Autodesk Inventor part; units mm, degrees
ref_plane "YZ Plane" through (0, 0, 0) normal (1, 0, 0) x (0, 1, 0)
ref_plane "XZ Plane" through (0, 0, 0) normal (0, 1, 0) x (-1, 0, 0)
ref_plane "XY Plane" through (0, 0, 0) normal (0, 0, 1) x (1, 0, 0)
sketch "Sketch1" plane through (0, 0, 0) normal (0, 1, 0) x (-1, 0, 0)
  line L0 (75, 0) -> (-75, 0)
  line L1 (-75, 0) -> (-75, -90)
  line L2 (-75, -90) -> (75, -90)
  line L3 (75, -90) -> (75, 0)
  point P0 (0, 0)
  point P1 (0, 0)
  dimension "d0" = 150
  dimension "d1" = 90
extrude "Extrusion1" add sketch "Sketch1" along normal blind 19
sketch "Sketch2" plane through (-75, 0, 0) normal (0, 0, 1) x (1, 0, 0)
  line L0 (0, 0) -> (150, 0)
  line L1 (150, 0) -> (150, 19)
  line L2 (0, 19) -> (150, 19)
  line L3 (0, 0) -> (0, 19)
  point P0 (75, 0)
  point P1 (75, 4)
  point P2 (75, 14)
  dimension "d4" = 4
  dimension "d5" = 14
  dimension "d6" = 75
  dimension "d7" = 75
hole "Hole1" at (0, 4, 0) at (0, 14, 0) direction (0, 0, -1) diameter 3.302 depth 21
sketch "Sketch3" plane through (0, 19, 0) normal (0, 1, 0) x (1, 0, 0)
  line L0 (-75, 0) -> (75, 0)
  line L1 (75, 0) -> (75, 90)
  line L2 (75, 90) -> (-75, 90)
  line L3 (-75, 90) -> (-75, 0)
  point P0 (0, 0)
  point P1 (-71.5, 85.914)
  point P2 (71.5, 85.914)
  point P3 (51.5, 3)
  point P4 (-51.5, 3)
  dimension "d15" = 143
  dimension "d16" = 4.086
  dimension "d17" = 3.5
  dimension "d18" = 4.086
  dimension "d20" = 23.5
  dimension "d21" = 3
  dimension "d22" = 3
  dimension "d39" = 23.5
hole "Hole2" at (-71.5, 19, -85.914) at (71.5, 19, -85.914) at (51.5, 19, -3) at (-51.5, 19, -3) direction (0, -1, 0) diameter 2.459 depth 18.535
properties part number "Bas"
The listing builds one solid part. Answer for the finished solid, in the listing's coordinates (mm). A direction names the side the tool comes from. Give positions to 0.01 mm unless a question says otherwise; leave off trailing zeros. Order: outer loops, then holes, each group sorted by start corner. A loop starts at its lowest first (then second) coordinate and runs counter-clockwise, first axis right, second up. Notation, with made-up numbers: (21.5, -6.75) - (46.5, -6.75) arc R16 ccw to (46.5, 1.25) - close; hole circle Ø4 at (-22.5, 87). An arc over 180 degrees is marked (long way). Use one line per item in the form item = value. Start each with the question number.
(1) The mould has two halves that part along Z. Classify faces 3 (the flat face through (-75, 9, -46)), 4 (the flat face through (1, 9, -90)), 5 (the flat face through (-1, 9, 0)): released by +Z, released by -Z, zero draft, split by the parting line, or undercut.
(2) A cutting plane is placed at A-A, the plane x = 0. Write down the section's boundary in (y, z), then the cut area to 3 significant figures.
(3) Consider line 1 (Y direction, x = 0, z = -15); line 2 (X direction, y = 4, z = -14.5); line 3 (Y direction, x = -1.5, z = -18). Determine where each line is inside the solid, lowest interval first. Write a range as from..to.
(4) Flat-ended cylindrical pins translate along their axes: pin 1 Ø0.7 at (x, z) = (52, -3) entering from +Y (3 decimals); pin 2 Ø3 at (x, y) = (0, 4) entering from +Z. Find the tip coordinate at first contact, or state that the pin passes through.
(5) For faces 1 (the cylindrical face through (-0.496, 12.425, -10.647)), 2 (the flat face through (1, 0, -44)), determine the directions among +Z, -Z, +X, -X, +Y, -Y from which every point of the face is accessible in a straight line to the end or side of a thin tool.
Ans:
q1.face_3 = zero draft
q1.face_4 = released by -Z
q1.face_5 = released by +Z
q2.outline = (0, -90) - (19, -90) - (19, 0) - (15.65, 0) - (15.65, -21) - (12.35, -21) - (12.35, 0) - (5.65, 0) - (5.65, -21) - (2.35, -21) - (2.35, 0) - (0, 0) - close
q2.area = 1,570 mm^2
q3.line_1 = 0..2.35, 5.65..12.35, 15.65..19
q3.line_2 = -75..-1.65, 1.65..75
q3.line_3 = 0..3.31, 4.69..13.31, 14.69..19
q4.pin_1 = 0.465
q4.pin_2 = -21
q5.face_1 = +Z
q5.face_2 = +Z, -Z, +X, -X, -Y
